Build history of the part. All positions in model axes, mm. A direction names the side the tool comes from. Give positions to 0.01 mm unless a question says otherwise; leave off trailing zeros. Order: outer loops, then holes, each group sorted by start corner. A loop starts at its lowest first (then second) coordinate and runs counter-clockwise, first axis right, second up. Notation, with made-up numbers: (2.5, 25) - (25.5, 25) arc R32 cw to (25.5, 54) - close; hole circle Ø7 at (2.25, 39.25). An arc over 180 degrees is marked (long way). Write each question's results on one line, items separated by ' | '. Start each with the question number.
from build123d import *

# Parameters (mm, degrees)
F0_W            = 210
F0_H            = 225
F1_DEPTH        = 25
F3_DEPTH        = 95
F4_R            = 37.5
F5_DEPTH        = 10
F5_DEPTH_BACK   = 127
F7_DEPTH        = 10
F7_DEPTH_BACK   = 127
F8_W            = 60
F8_H            = 60
F9_DEPTH        = 10
F10_R           = 10
F12_DEPTH       = 20
F14_D           = 15
F14_CBORE_D     = 30
F14_CBORE_DEPTH = 10
F15_R           = 10
F16_R           = 18.1648840972
F17_DEPTH       = 235.001
F18_R           = 19.5
F19_DEPTH       = 220.001
F20_SIZE        = 2
F21_R           = 10


with BuildPart() as f1:
    # F0 (on Top) → F1 (new body)
    with BuildSketch(Plane.XY):
        Rectangle(F0_W, F0_H)
    extrude(amount=F1_DEPTH)

    # F2 (on face) → F3 (join)
    with BuildSketch(Plane.XY.offset(25)):
        with BuildLine():
            Line((-71, -32.5), (-71, -112.5))
            Line((-71, -112.5), (-56, -112.5))
            Line((-56, -112.5), (-56, -46.4818166789))
            ThreePointArc((-56, -46.4818166789), (7.4888527117, -14.9888527117), (38.9818166789, 48.5))
            Line((38.9818166789, 48.5), (105, 48.5))
            Line((105, 48.5), (105, 63.5))
            Line((105, 63.5), (25, 63.5))
            ThreePointArc((25, 63.5), (-3.1177490061, -4.3822509939), (-71, -32.5))
        make_face()
    extrude(amount=F3_DEPTH)

    # F4 (on face) → F5 (join, two sides)
    with BuildSketch(Plane.XZ.offset(112.5)) as f5_sk:
        with Locations((-63.5, 120)):
            Circle(F4_R)
    extrude(amount=F5_DEPTH)
    extrude(f5_sk.sketch, amount=-F5_DEPTH_BACK)

    # F6 (on face) → F7 (join, two sides)
    with BuildSketch(Plane.YZ.offset(105)) as f7_sk:
        with BuildLine():
            ThreePointArc((63.5, 80.7094158862), (86.8220700148, 94.504902432), (96, 120))
            ThreePointArc((96, 120), (30.504902432, 150.8220700148), (48.5, 80.7094158862))
            Line((48.5, 80.7094158862), (48.5, 120))
            Line((48.5, 120), (63.5, 120))
            Line((63.5, 120), (63.5, 80.7094158862))
        make_face()
        with BuildLine():
            Line((48.5, 120), (48.5, 80.7094158862))
            ThreePointArc((48.5, 80.7094158862), (56, 80), (63.5, 80.7094158862))
            Line((63.5, 80.7094158862), (63.5, 120))
            Line((63.5, 120), (48.5, 120))
        make_face()
    extrude(amount=F7_DEPTH)
    extrude(f7_sk.sketch, amount=-F7_DEPTH_BACK)

    # F8 (on face) → F9 (join)
    with BuildSketch(Plane.XY.offset(25)):
        with Locations((75, -82.5)):
            Rectangle(F8_W, F8_H)
    extrude(amount=F9_DEPTH)

    # F10
    f10_edges = [f1.edges().sort_by_distance(p)[0] for p in [
        (45, -52.5, 30),
    ]]
    fillet(f10_edges, radius=F10_R)

    # F11 (on face) → F12 (cut)
    with BuildSketch(Plane.XY.offset(25)):
        with BuildLine():
            ThreePointArc((46.5755076536, 39.5), (13.8528137424, -21.3528137424), (-47, -54.0755076536))
            Line((-47, -54.0755076536), (-47, -103.5))
            Line((-47, -103.5), (36, -103.5))
            Line((36, -103.5), (36, -62.5))
            ThreePointArc((36, -62.5), (41.5649711575, -49.0649711575), (55, -43.5))
            Line((55, -43.5), (96, -43.5))
            Line((96, -43.5), (96, 39.5))
            Line((96, 39.5), (46.5755076536, 39.5))
        make_face()
    extrude(amount=-F12_DEPTH, mode=Mode.SUBTRACT)

    # F14 (through all)
    with Locations(Plane.XY.offset(35)):
        with Locations((75, -82.5)):
            CounterBoreHole(F14_D / 2, F14_CBORE_D / 2, F14_CBORE_DEPTH)

    # F15
    f15_edges = [f1.edges().sort_by_distance(p)[0] for p in [
        (-47, -54.075508, 15),
        (-47, -103.5, 15),
        (46.575508, 39.5, 15),
        (96, 39.5, 15),
        (96, -43.5, 15),
        (36, -103.5, 15),
    ]]
    fillet(f15_edges, radius=F15_R)

    # F16 (on face) → F17 (cut, through all)
    with BuildSketch(Plane.XZ.offset(122.5)):
        with Locations((-63.5, 120)):
            Circle(F16_R)
    extrude(amount=-F17_DEPTH, mode=Mode.SUBTRACT)

    # F18 (on face) → F19 (cut, through all)
    with BuildSketch(Plane.YZ.offset(115)):
        with Locations((56, 120)):
            Circle(F18_R)
    extrude(amount=-F19_DEPTH, mode=Mode.SUBTRACT)

    # F20
    f20_edges = [f1.edges().sort_by_distance(p)[0] for p in [
        (-81.664884, -122.5, 120),
        (115, 36.5, 120),
        (-81.664884, 14.5, 120),
        (-22, 36.5, 120),
    ]]
    chamfer(f20_edges, length=F20_SIZE)

    # F21
    f21_edges = [f1.edges().sort_by_distance(p)[0] for p in [
        (105, -112.5, 17.5),
        (105, 112.5, 12.5),
        (-105, 112.5, 12.5),
        (-105, -112.5, 12.5),
    ]]
    fillet(f21_edges, radius=F21_R)


solid = f1.part
Item 1: Flat gauge pins, fed straight in: pin 1 Ø1.5 at (x, y) = (68, 33) entering from +Z; pin 2 Ø9 at (x, y) = (71.5, -88.5) entering from +Z; pin 3 Ø3 at (x, z) = (22, 131.5) entering from -Y; pin 4 Ø3 at (y, z) = (46.5, 138) entering from +X. Where does each tip first touch, or does it go through?
Item 2: Cut at B-B, the plane x = 75. List the corners of the cut face in (y, z), then the cut area to 3 significant figures.
Item 3: Cut at D-D, the plane y = 56. List the corners of the cut face in (x, z), then the cut area to 3 significant figures.
Item 4: Two-plate mould, pull along Y, no slides. Class faces 4 (the flat face through (70, -43.5, 15)), 5 (the flat face through (105, 0, 22)), 6 (the flat face through (-1, 112.5, 12)): +Y half, -Y half, draft (parallel to the pull), parting line (faces both ways), or undercut.
Item 5: Cut at C-C, the plane y = -82.5. List the corners of the cut face in (x, z).
Item 6: Probe line 1 along Y through (x, z) = (75, 20); line 2 along Y through (x, z) = (75, 32.5); line 3 along Z through (x, y) = (68.5, 56). List the from-to ranges inside material, lowest first. Write a range as from..to.
Item 7: Cut at A-A, the plane z = 28.5. List the corners of the cut face in (x, y).
Item 8: Which spindle directions (+Z, -Z, +X, -X, +Y, -Y) get a long thin tool onto all of the face, cutting with end or side? Do faces 1 (the flat face through (-56, -80, 54)), 2 (the cylindrical face through (48.33, 37.39, 14.86)), 3 (the cylindrical face through (32.99, -100.65, 14.86)). Say none if no direction does.
Values found:
1) pin 1: stops at z = 153.24 | pin 2: stops at z = 25 | pin 3: stops at y = 17.27 | pin 4: stops at x = 115
2) outline: (-112.5, 0) - (-90, 0) - (-90, 25) - (-97.5, 25) - (-97.5, 35) - (-112.5, 35) - close; (-75, 0) - (112.5, 0) - (112.5, 25) - (63.5, 25) - (63.5, 80.71) arc R40 ccw (long way) to (48.5, 80.71) - (48.5, 25) - (39.5, 25) - (39.5, 5) - (-43.5, 5) - (-43.5, 25) - (-52.5, 25) - (-52.5, 35) - (-67.5, 35) - (-67.5, 25) - (-75, 25) - close; hole circle Ø39 at (56, 120) | area: 8,550 mm2
3) outline: (-105, 0) - (105, 0) - (105, 80) - (115, 80) - (115, 98.5) - (113, 100.5) - (-20, 100.5) - (-22, 98.5) - (-22, 80) - (24.71, 80) - (24.71, 25) - (-105, 25) - close; (-22, 141.5) - (-20, 139.5) - (113, 139.5) - (115, 141.5) - (115, 160) - (-22, 160) - close | area: 15,300 mm2
4) face 4: undercut | face 5: draft | face 6: +Y half
5) outline: (-105, 0) - (67.5, 0) - (67.5, 25) - (60, 25) - (60, 35) - (45, 35) - (45, 25) - (36, 25) - (36, 5) - (-47, 5) - (-47, 25) - (-56, 25) - (-56, 83.26) arc R37.5 ccw (long way) to (-71, 83.26) - (-71, 25) - (-105, 25) - close; (82.5, 0) - (105, 0) - (105, 35) - (90, 35) - (90, 25) - (82.5, 25) - close; hole circle Ø36.33 at (-63.5, 120)
6) line 1: y = -112.5..-90, -75..-43.5, 39.5..112.5 | line 2: y = -112.5..-97.5, -67.5..-52.5, 48.5..63.5 | line 3: z = 0..100.5, 139.5..160
7) outline: (-71, -112.5) - (-56, -112.5) - (-56, -46.48) arc R111 ccw to (38.98, 48.5) - (105, 48.5) - (105, 63.5) - (25, 63.5) arc R96 cw to (-71, -32.5) - close; (45, -112.5) - (95, -112.5) arc R10 ccw to (105, -102.5) - (105, -52.5) - (55, -52.5) arc R10 ccw to (45, -62.5) - close; hole circle Ø30 at (75, -82.5)
8) face 1: -Y | face 2: none | face 3: +Z
